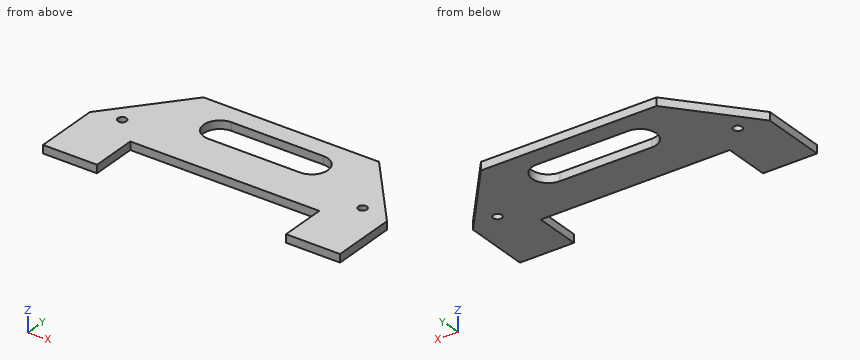
from build123d import *

# Parameters (mm, degrees)
SALIENTE_EXTRUIR1_DEPTH          = 3
TALADRO_DE_MARGEN_PARA_M31_D     = 3.2
TALADRO_DE_MARGEN_PARA_M31_DEPTH = 5
TALADRO_DE_MARGEN_PARA_M31_TIP   = 0.96137699
CORTAR_EXTRUIR1_REACH            = 77.067
CROQUIS4_W                       = 70
CROQUIS4_H                       = 17
CORTAR_EXTRUIR2_REACH            = 77.067


with BuildPart() as part:
    # Croquis1 → Saliente-Extruir1 (new body)
    with BuildSketch(Plane.XY):
        Polygon((-55, 0), (55, 0), (55, 24), (32.5, 51), (-32.5, 51), (-55, 24), align=None)
    extrude(amount=SALIENTE_EXTRUIR1_DEPTH)

    # Taladro de margen para M31
    with Locations(Plane(origin=(44.5, 26, 0), x_dir=(-1, 0, 0), z_dir=(0, 0, -1))):
        with Locations((0, 0), (89, 0)):
            Hole(TALADRO_DE_MARGEN_PARA_M31_D / 2, depth=TALADRO_DE_MARGEN_PARA_M31_DEPTH)
            with Locations((0, 0, -(TALADRO_DE_MARGEN_PARA_M31_DEPTH + TALADRO_DE_MARGEN_PARA_M31_TIP / 2))):  # 118° drill point
                Cone(0, TALADRO_DE_MARGEN_PARA_M31_D / 2, TALADRO_DE_MARGEN_PARA_M31_TIP, mode=Mode.SUBTRACT)

    # Croquis4 → Cortar-Extruir1 (cut, up to next)
    with BuildSketch(Plane.XY.offset(3), mode=Mode.PRIVATE) as cortar_extruir1_sk1:
        with Locations((0, 8.5)):
            Rectangle(CROQUIS4_W, CROQUIS4_H)
    cortar_extruir1_tool1 = extrude(cortar_extruir1_sk1.sketch, amount=-CORTAR_EXTRUIR1_REACH, mode=Mode.PRIVATE) & part.part
    add(cortar_extruir1_tool1.solids().sort_by_distance((0, 8.5, 3))[0], mode=Mode.SUBTRACT)

    # Croquis5 → Cortar-Extruir2 (cut, up to next)
    with BuildSketch(Plane.XY.offset(3), mode=Mode.PRIVATE) as cortar_extruir2_sk1:
        with BuildLine():
            Line((-17, 44), (17, 44))
            ThreePointArc((17, 44), (23, 38), (17, 32))
            Line((17, 32), (-17, 32))
            ThreePointArc((-17, 32), (-23, 38), (-17, 44))
        make_face()
    cortar_extruir2_tool1 = extrude(cortar_extruir2_sk1.sketch, amount=-CORTAR_EXTRUIR2_REACH, mode=Mode.PRIVATE) & part.part
    add(cortar_extruir2_tool1.solids().sort_by_distance((0, 38, 3))[0], mode=Mode.SUBTRACT)


solid = part.part
Geometry: final body of the model. Coordinates: model frame, mm. Coordinates: 2 decimals unless noted, no trailing zeros. Loops run counter-clockwise (first coordinate to the right, second up) from the corner with the lowest first, then second, coordinate; pieces in that order, holes last. Notation, with made-up numbers: (21.25, 72.5) - (64.25, 72.5) arc R11 cw to (64.25, 88.5) - close; hole circle Ø10 at (76, 29). An arc over 180 degrees is marked (long way). Put each result on its own line as item: value. Start each with the question number.
Q1. Line query: line 1 (Y direction, x = 8, z = 1.3); line 2 (X direction, y = 11.5, z = 2.7); line 3 (Y direction, x = 44.5, z = 2.2). Output: solid intervals per line, ascending.
Q2. Cut plane B-B, the plane x = -44.5. Return loops of the section in (y, z).
Q3. Cut plane C-C, the plane y = 8. Return loops of the section in (x, z).
Q4. Pin query (flat end, axial travel): pin 1 Ø6 at (x, y) = (8, 21) entering from -Z; pin 2 Ø0.9 at (x, z) = (2.5, 1.5) entering from -Y. Return the tip coordinate at first contact, or that it passes through.
Q5. Cut plane D-D, the plane y = 26. Return loops of the section in (x, z).
Q6. Cut plane A-A, the plane z = 1.6. Return loops of the section in (x, y).
Filled sheet:
1. line 1: 17 to 32, 44 to 51
1. line 2: -55 to -35, 35 to 55
1. line 3: 0 to 24.4, 27.6 to 36.6
2. outline: (0, 0) - (24.4, 0) - (24.4, 3) - (0, 3) - close; (27.6, 0) - (36.6, 0) - (36.6, 3) - (27.6, 3) - close
3. outline: (-55, 0) - (-35, 0) - (-35, 3) - (-55, 3) - close; (35, 0) - (55, 0) - (55, 3) - (35, 3) - close
4. pin 1: z = 0
4. pin 2: y = 17
5. outline: (-53.33, 0) - (-46.1, 0) - (-46.1, 3) - (-53.33, 3) - close; (-42.9, 0) - (42.9, 0) - (42.9, 3) - (-42.9, 3) - close; (46.1, 0) - (53.33, 0) - (53.33, 3) - (46.1, 3) - close
6. outline: (-55, 0) - (-35, 0) - (-35, 17) - (35, 17) - (35, 0) - (55, 0) - (55, 24) - (32.5, 51) - (-32.5, 51) - (-55, 24) - close; hole circle Ø3.2 at (-44.5, 26); hole (-17, 32) - (17, 32) arc R6 ccw to (17, 44) - (-17, 44) arc R6 ccw to start; hole circle Ø3.2 at (44.5, 26)
